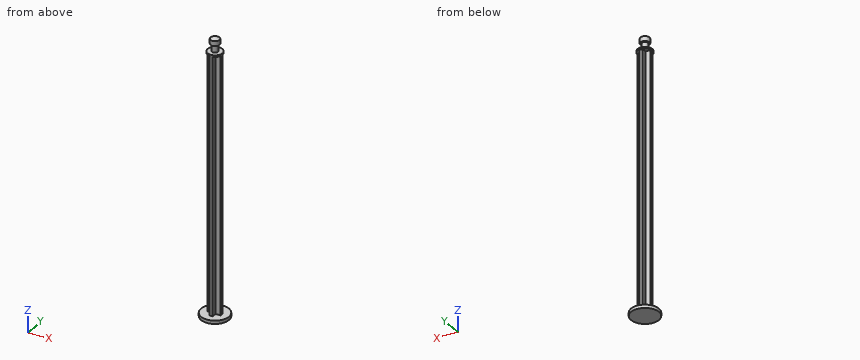
from build123d import *

# Parameters (mm, degrees)
AUFSATZ_LINEAR_AUSTRAGEN1_DEPTH = 78
SKIZZE3_R                       = 4.25
AUFSATZ_LINEAR_AUSTRAGEN3_DEPTH = 1
FASE1_SIZE2                     = 1.375
FASE1_SIZE                      = 0.500459072


with BuildPart() as part:
    # Skizze1 → Aufsatz-Linear austragen1 (new body)
    with BuildSketch(Plane.XY):
        Polygon((0.5, 0.5), (2, 0.5), (2, -0.5), (0.5, -0.5), (0.5, -2), (-0.5, -2), (-0.5, -0.5), (-2, -0.5), (-2, 0.5), (-0.5, 0.5), (-0.5, 2), (0.5, 2), align=None)
    extrude(amount=AUFSATZ_LINEAR_AUSTRAGEN1_DEPTH)

    # Skizze3 → Aufsatz-Linear austragen3 (add)
    with BuildSketch(Plane(origin=(0, 0, 0), x_dir=(-1, 0, 0), z_dir=(0, 0, -1))):
        Circle(SKIZZE3_R)
    extrude(amount=AUFSATZ_LINEAR_AUSTRAGEN3_DEPTH)

    # Skizze4 → Rotation1 (revolve)
    with BuildSketch(Plane(origin=(0, 0, 0), x_dir=(0, 0, -1), z_dir=(1, 0, 0))):
        Polygon((-78, 0), (-78, 1.335941473), (-78, 2.25), (-78.5, 2.25), (-78.5, 0.875), (-80.75, 0.875), (-80.75, 1.375), (-82.75, 1.375), (-82.75, 0), align=None)
    revolve(axis=Axis((0, 0, 0), (0, 0, 1)))

    # Fase1
    fase1_edges = [part.edges().sort_by_distance(p)[0] for p in [
        (0, -1.375, 82.75),
    ]]
    fase1_side = [part.faces().sort_by_distance(p)[0] for p in [
        (0, -1.375, 82.739990819),
    ]]
    chamfer(fase1_edges, length=FASE1_SIZE - 0.0001, length2=FASE1_SIZE2 - 0.0001, reference=fase1_side[0])  # a hair under: the kernel refuses the full size


solid = part.part
The listing builds one solid part. Answer for the finished solid, in the listing's coordinates (mm). Round coordinates to 2 decimals unless told otherwise and drop trailing zeros. Order: outer loops, then holes, each group sorted by start corner. A loop starts at its lowest first (then second) coordinate and runs counter-clockwise, first axis right, second up. Notation, with made-up numbers: (72, 16) -> (84, 16) arc R19 ccw to (84, 38) -> close; hole circle Ø11 at (11, 61.5). An arc over 180 degrees is marked (long way). One line per item, written item: value.
Item 1: Straight lines are drawn through the part: L1, parallel to Z at x = -1.25, y = -2.75; L2, parallel to Y at x = -1.75, z = 8. For each, find the intervals that lie inside material, in ascending order.
Taken from the geometry:
L1: z = -1 to 0
L2: y = -0.5 to 0.5
Item 2: Find section A-A, the plane z = 41. Give the vertices of the cut face in (x, y).
Taken from the geometry:
outline: (-2, -0.5) -> (-0.5, -0.5) -> (-0.5, -2) -> (0.5, -2) -> (0.5, -0.5) -> (2, -0.5) -> (2, 0.5) -> (0.5, 0.5) -> (0.5, 2) -> (-0.5, 2) -> (-0.5, 0.5) -> (-2, 0.5) -> close
Item 3: Given P1, Ø1.1, axis at x = 0, z = 45, coming from the +Y side; P2, Ø4, axis at x = 0.5, z = 18.5, coming from the -Y side; P3, Ø1.6, axis at x = -1.5, z = 35, coming from the -Y side, each flat-ended and moving along its own axis, determine where each tip first touches the part or whether it passes through.
Taken from the geometry:
P1: stops at y = 2
P2: stops at y = -2
P3: stops at y = -0.5
Item 4: Find section C-C, the plane x = -3.5. Give the vertices of the cut face in (y, z).
Taken from the geometry:
outline: (-2.41, -1) -> (2.41, -1) -> (2.41, 0) -> (-2.41, 0) -> close
Item 5: Find section B-B, the plane y = 3. Give the vertices of the cut face in (x, z), then the cut area to 3 significant figures.
Taken from the geometry:
outline: (-3.01, -1) -> (3.01, -1) -> (3.01, 0) -> (-3.01, 0) -> close
area: 6.02 mm2
